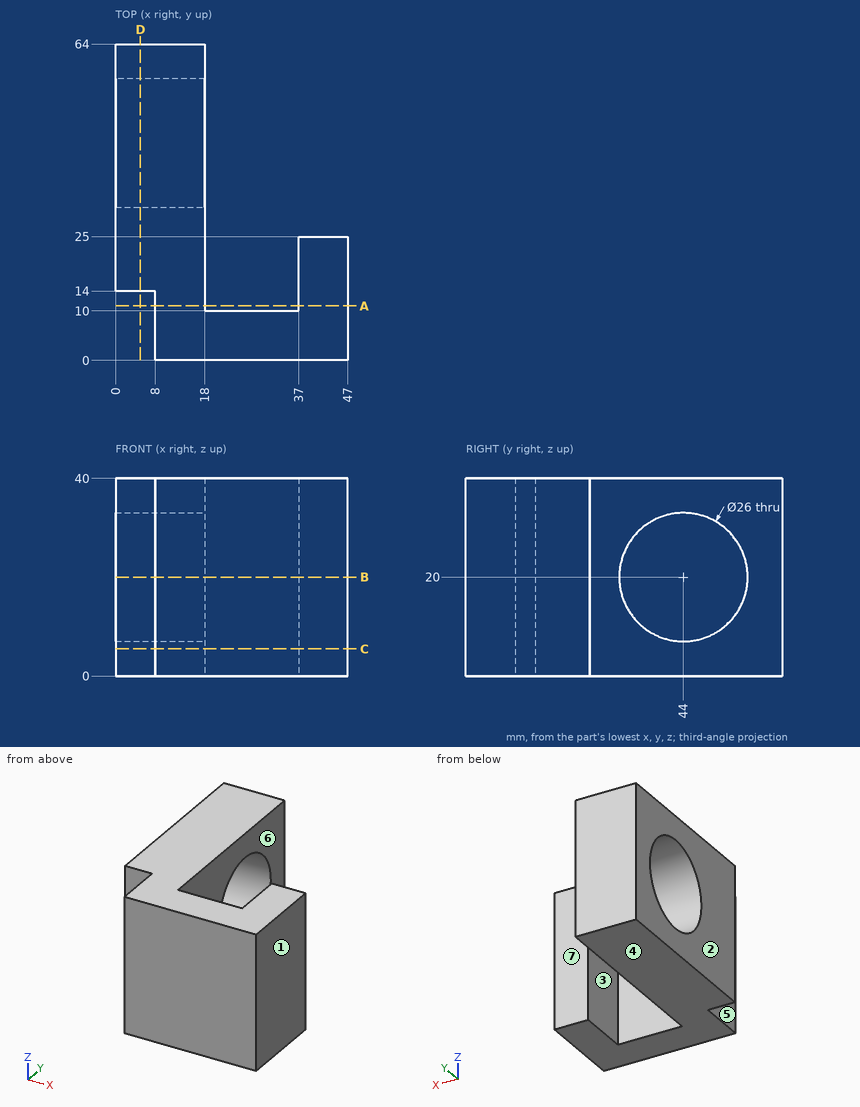
Check sheet for the drawn part. Datum: minimum x, y, z corner. Units: mm. A direction names the side the tool comes from. Give positions to 0.01 mm unless a question says otherwise; leave off trailing zeros. Order: outer loops, then holes, each group sorted by start corner. A loop starts at its lowest first (then second) coordinate and runs counter-clockwise, first axis right, second up. Notation, with made-up numbers: (12.5, 67) - (30.5, 67) arc R30 ccw to (30.5, 89) - close; hole circle Ø9 at (-24.5, -36.75). An arc over 180 degrees is marked (long way). Write item = value, one per line. Start each with the question number.
1) Draft check along X on the marked faces 1, 2 and 3. Enter one of: released by +X, released by -X, zero draft, split by the parting line, or undercut.
2) Section check B-B (z = 20). Enter the section's corners in (x, y), then the cut area to 3 significant figures.
3) Scan lines: L1, parallel to X at y = 20, z = 37; L2, parallel to Z at x = 4, y = 44; L3, parallel to Y at x = 36.5, z = 24. Record each from-to range of solid material in increasing order.
4) Section check C-C (z = 5.5). Enter the section's corners in (x, y), then the cut area to 3 significant figures.
5) Section check D-D (x = 5). Enter the section's corners in (y, z), then the cut area to 3 significant figures.
6) Section check A-A (y = 11). Enter the section's corners in (x, z).
7) Gauge pin test, flat ends, axial feed: pin 1 Ø2.5 at (x, z) = (5.5, 25.5) entering from -Y; pin 2 Ø4 at (x, z) = (39.5, 8.5) entering from +Y; pin 3 Ø4 at (y, z) = (32.5, 12.5) entering from +X; pin 4 Ø4 at (y, z) = (35, 26) entering from +X. Record the tip position at first contact, or that the pin passes through.
8) Access from +Z, -Z, +X, -X, +Y, -Y to the whole of each face (thin tool, end or side, straight path). Record for the marked faces 4, 5, 6 and 7.
Geometry check:
q1.face_1 = released by +X
q1.face_2 = released by -X
q1.face_3 = undercut
q2.outline = (0, 14) - (8, 14) - (8, 0) - (47, 0) - (47, 25) - (37, 25) - (37, 10) - (18, 10) - (18, 31) - (0, 31) - close; (0, 57) - (18, 57) - (18, 64) - (0, 64) - close
q2.area = 1,010 mm2
q3.L1 = 0 to 18, 37 to 47
q3.L2 = 0 to 7, 33 to 40
q3.L3 = 0 to 10
q4.outline = (0, 14) - (8, 14) - (8, 0) - (47, 0) - (47, 25) - (37, 25) - (37, 10) - (18, 10) - (18, 64) - (0, 64) - close
q4.area = 1,480 mm2
q5.outline = (14, 0) - (64, 0) - (64, 40) - (14, 40) - close; hole circle Ø26 at (44, 20)
q5.area = 1,470 mm2
q6.outline = (8, 0) - (18, 0) - (18, 40) - (8, 40) - close; (37, 0) - (47, 0) - (47, 40) - (37, 40) - close
q7.pin_1 = 14
q7.pin_2 = 25
q7.pin_3 = 18
q7.pin_4 = through
q8.face_4 = -Z, +X, -X, +Y, -Y
q8.face_5 = +Z, -Z, -X, -Y
q8.face_6 = +Z, -Z, +Y
q8.face_7 = +Z, -Z, +X, +Y
